The model under review builds one solid part; all positions refer to its coordinate system, in mm. A direction names the side the tool comes from. Coordinates: 2 decimals unless noted, no trailing zeros. Write each loop counter-clockwise with the first axis right and the second up, starting at its lowest first coordinate (ties: lowest second). Pieces come first, ordered by that corner, then holes. Notation, with made-up numbers: (-32.75, 86.5) - (21.25, 86.5) arc R9 cw to (21.25, 100.5) - close; hole circle Ø4 at (-25.5, 8.25). An arc over 180 degrees is marked (long way). Return JSON: item names as keys, results as strings. Group by question number.
(1) We need section A-A on x = 0. State the section outline as (y, z) points, then the cut area to 3 significant figures.
(2) To check wall thickness, follow L1, parallel to Z at x = -7.75, y = -14.75; L2, parallel to Y at x = 7.5, z = 15; L3, parallel to Z at x = 15.5, y = -12.25. State the ranges of each line that lie inside material, in increasing order. Write a range as from..to.
(3) We need section C-C on z = -9. State the section outline as (x, y) points, then the cut area to 3 significant figures.
(4) We need section D-D on y = -30. State the section outline as (x, z) points.
(5) For pin 1 Ø1 at (y, z) = (-25, 12) entering from -X; pin 2 Ø1 at (x, y) = (-0.5, 1) entering from -Z; pin 3 Ø4 at (x, z) = (-15.5, 0) entering from +Y, all flat-tipped, find the tip position at first contact; note any pin that passes through.
(6) Draft analysis for pull direction X (two halves, no side actions). For faces 1 (the face through (3, -4.496, 8)), 2 (the face through (0.264, -7.031, 0.756)), 3 (the face through (15.7, -18.62, 0.08)), state which applies: released by +X, released by -X, zero draft, split by the parting line, or undercut.
(7) Tool access review of faces 4 (the face through (-6.83, -13.81, -14.27)), 5 (the face through (5.407, -43.856, -17.169)), 6 (the face through (0, 4, 4.25)): name each direction out of +Z, -Z, +X, -X, +Y, -Y from which nothing blocks a thin tool from reaching the whole face with its end or side.
(8) We need section B-B on y = -13. State the section outline as (x, z) points, then the cut area to 3 significant figures.
```python
from build123d import *

# Parameters (mm, degrees)
SKETCH_1_W                  = 18.5
SKETCH_1_H                  = 24.5
SKETCH_2_R                  = 6
EXTRUDE_1_DEPTH             = 5
SKETCH_3_R                  = 3
EXTRUDE_2_DEPTH             = 15.5
CUT_EXTRUDE_START           = -14
CUT_EXTRUDE_1_DEPTH         = 14
SKETCH_5_R                  = 18
EXTRUDE_3_DEPTH             = 20
HOLE_WIZARD_2_5_2_5_1_D     = 2.5
HOLE_WIZARD_2_5_2_5_1_DEPTH = 8.5
HOLE_WIZARD_2_5_2_5_1_TIP   = 0.751075774


with BuildPart() as part:
    # 草图1 → 旋转1 (revolve)
    with BuildSketch(Plane(origin=(0, 0, 0), x_dir=(-1, 0, 0), z_dir=(0, 0, -1)), mode=Mode.PRIVATE) as revolve_1_sk:
        with Locations((-9.25, -21.746377743)):
            Rectangle(SKETCH_1_W, SKETCH_1_H)
    revolve(revolve_1_sk.sketch.rotate(Axis((0, -33.996377743, 0), (0, 1, 0)), 270), axis=Axis((0, -33.996377743, 0), (0, 1, 0)))

    # 草图2 → 凸台-拉伸1 (add)
    with BuildSketch(Plane(origin=(0, -9.496377743, 0), x_dir=(-1, 0, 0), z_dir=(0, 1, 0))):
        with Locations(Location((0, 6.75, 0), (0, 0, 90))):
            Circle(SKETCH_2_R)
    extrude(amount=EXTRUDE_1_DEPTH)

    # 草图3 → 凸台-拉伸2 (add)
    with BuildSketch(Plane(origin=(0, -4.496377743, 0), x_dir=(-1, 0, 0), z_dir=(0, 1, 0))):
        with Locations(Location((0, 6.75, 0), (0, 0, 90))):
            Circle(SKETCH_3_R)
    extrude(amount=EXTRUDE_2_DEPTH)

    # 草图4 → 切除-拉伸1 (cut)
    with BuildSketch(Plane(origin=(0, 11.003622257, 0), x_dir=(-1, 0, 0), z_dir=(0, 1, 0)).offset(CUT_EXTRUDE_START)):
        with BuildLine():
            Line((1.658312395, 4.25), (-1.658312395, 4.25))
            ThreePointArc((-1.658312395, 4.25), (0, 3.75), (1.658312395, 4.25))
        make_face()
    extrude(amount=CUT_EXTRUDE_1_DEPTH, mode=Mode.SUBTRACT)

    # 草图5 → 凸台-拉伸3 (add)
    with BuildSketch(Plane.XZ.offset(33.996377743)):
        with Locations(Location((0, 0, 0), (0, 0, 270))):
            Circle(SKETCH_5_R)
    extrude(amount=EXTRUDE_3_DEPTH)

    # Ø2.5 (2.5) 直径孔1
    with Locations(Plane(origin=(0, -9.496377743, 0), x_dir=(1, 0, 0), z_dir=(0, 1, 0))):
        with Locations((-7.75, 13.423393759), (7.75, 13.423393759), (15.5, 0), (7.75, -13.423393759), (-7.75, -13.423393759), (-15.5, 0)):
            Hole(HOLE_WIZARD_2_5_2_5_1_D / 2, depth=HOLE_WIZARD_2_5_2_5_1_DEPTH)
            with Locations((0, 0, -(HOLE_WIZARD_2_5_2_5_1_DEPTH + HOLE_WIZARD_2_5_2_5_1_TIP / 2))):  # 118° drill point
                Cone(0, HOLE_WIZARD_2_5_2_5_1_D / 2, HOLE_WIZARD_2_5_2_5_1_TIP, mode=Mode.SUBTRACT)


solid = part.part
```
Ans:
{
 "1": {"outline": "(-54, -18) - (-34, -18) - (-34, -18.5) - (-9.5, -18.5) - (-9.5, 0.75) - (-4.5, 0.75) - (-4.5, 3.75) - (-3, 3.75) - (-3, 4.25) - (11, 4.25) - (11, 9.75) - (-4.5, 9.75) - (-4.5, 12.75) - (-9.5, 12.75) - (-9.5, 18.5) - (-34, 18.5) - (-34, 18) - (-54, 18) - close", "area": "1,770 mm²"},
 "2": {"L1": "-16.8..-14.67, -12.17..12.17, 14.67..16.8", "L2": "-54..-9.5", "L3": "-10.1..-1.25, 1.25..10.1"},
 "3": {"outline": "(-16.16, -34) - (-15.59, -34) - (-15.59, -54) - (15.59, -54) - (15.59, -34) - (16.16, -34) - (16.16, -9.5) - (-16.16, -9.5) - close", "area": "1,420 mm²"},
 "4": {"outline": "circle Ø37 at (0, 0)"},
 "5": {"pin 1": "x = -14.49", "pin 2": "z = 4.25", "pin 3": "y = -9.5"},
 "6": {"face 1": "zero draft", "face 2": "split by the parting line", "face 3": "undercut"},
 "7": {"face 4": "+Y", "face 5": "-Y", "face 6": "-Z, +X, -X, +Y"},
 "8": {"outline": "circle Ø37 at (0, 0); hole circle Ø2.5 at (-15.5, 0); hole circle Ø2.5 at (-7.75, -13.42); hole circle Ø2.5 at (-7.75, 13.42); hole circle Ø2.5 at (7.75, -13.42); hole circle Ø2.5 at (7.75, 13.42); hole circle Ø2.5 at (15.5, 0)", "area": "1,050 mm²"}
}
